Source: CAD feature listing. Evaluate the final solid. Frame: model axes, mm. A direction names the side the tool comes from. Give positions to 0.01 mm unless a question says otherwise; leave off trailing zeros. Loops run counter-clockwise (first coordinate to the right, second up) from the corner with the lowest first, then second, coordinate; pieces in that order, holes last. Notation, with made-up numbers: M 18,65 L 41,65 A15 cw 41,75 Z; hole C -16.5,-4 d10. An arc over 180 degrees is marked long. Answer in a Markdown table with one row per item.
```python
from build123d import *

# Parameters (mm, degrees)
BOSS_EXTRUDE1_DEPTH      = 1.5875
BOSS_EXTRUDE1_DEPTH_BACK = 1.5875
SKETCH1_W                = 255.27
SKETCH1_H                = 73.96988
SKETCH1_R                = 1.5
BOSS_EXTRUDE2_DEPTH      = 1.5875
BOSS_EXTRUDE2_DEPTH_BACK = 1.5875
SKETCH1_4_W              = 255.27
SKETCH1_4_H              = 73.96988
CUT_EXTRUDE1_DEPTH       = 1.5875
CUT_EXTRUDE2_DEPTH       = 3.175
CUT_EXTRUDE2_DEPTH_BACK  = 3.175
SKETCH1_6_R              = 1.5
SKETCH3_R                = 1.5875
BOSS_EXTRUDE3_DEPTH      = 3.175


with BuildPart() as part:
    # Sketch1 → Boss-Extrude1 (new, two sides: drawn at the far end of the back side and taken through both)
    with BuildSketch(Plane(origin=(0, 0, 0), x_dir=(1, 0, 0), z_dir=(0, 1, 0)).offset(-BOSS_EXTRUDE1_DEPTH_BACK)):
        with Locations((127.635, 36.98494)):
            Rectangle(SKETCH1_W, SKETCH1_H)
        with Locations(Location((178.435, 68.57238, 0), (0, 0, 270))):
            Circle(SKETCH1_R, mode=Mode.SUBTRACT)
        with Locations(Location((178.435, 5.3975, 0), (0, 0, 270))):
            Circle(SKETCH1_R, mode=Mode.SUBTRACT)
        with Locations(Location((229.235, 68.57238, 0), (0, 0, 270))):
            Circle(SKETCH1_R, mode=Mode.SUBTRACT)
        with Locations(Location((229.235, 5.3975, 0), (0, 0, 270))):
            Circle(SKETCH1_R, mode=Mode.SUBTRACT)
        with Locations(Location((127.635, 68.57238, 0), (0, 0, 270))):
            Circle(SKETCH1_R, mode=Mode.SUBTRACT)
        with Locations(Location((127.635, 5.3975, 0), (0, 0, 270))):
            Circle(SKETCH1_R, mode=Mode.SUBTRACT)
        with Locations(Location((26.035, 5.3975, 0), (0, 0, 270))):
            Circle(SKETCH1_R, mode=Mode.SUBTRACT)
        with Locations(Location((76.835, 5.3975, 0), (0, 0, 270))):
            Circle(SKETCH1_R, mode=Mode.SUBTRACT)
        with Locations(Location((26.035, 68.57238, 0), (0, 0, 270))):
            Circle(SKETCH1_R, mode=Mode.SUBTRACT)
        with Locations(Location((76.835, 68.57238, 0), (0, 0, 270))):
            Circle(SKETCH1_R, mode=Mode.SUBTRACT)
    extrude(amount=BOSS_EXTRUDE1_DEPTH + BOSS_EXTRUDE1_DEPTH_BACK)

    # Sketch1_4 → Boss-Extrude2 (add, two sides: drawn at the far end of the back side and taken through both)
    with BuildSketch(Plane(origin=(0, 0, 0), x_dir=(1, 0, 0), z_dir=(0, 1, 0)).offset(-BOSS_EXTRUDE2_DEPTH_BACK)):
        with Locations((127.635, 36.98494)):
            Rectangle(SKETCH1_4_W, SKETCH1_4_H)
    extrude(amount=BOSS_EXTRUDE2_DEPTH + BOSS_EXTRUDE2_DEPTH_BACK)

    # Sketch2 → Cut-Extrude1 (cut)
    with BuildSketch(Plane(origin=(0, 1.5875, 0), x_dir=(1, 0, 0), z_dir=(0, 1, 0))):
        with BuildLine():
            Line((13.335, 63.80988), (241.935, 63.80988))
            ThreePointArc((241.935, 63.80988), (244.18006403, 62.87994403), (245.11, 60.63488))
            Line((245.11, 60.63488), (245.11, 13.335))
            ThreePointArc((245.11, 13.335), (244.18006403, 11.08993597), (241.935, 10.16))
            Line((241.935, 10.16), (13.335, 10.16))
            ThreePointArc((13.335, 10.16), (11.08993597, 11.08993597), (10.16, 13.335))
            Line((10.16, 13.335), (10.16, 60.63488))
            ThreePointArc((10.16, 60.63488), (11.08993597, 62.87994403), (13.335, 63.80988))
        make_face()
    extrude(amount=-CUT_EXTRUDE1_DEPTH, mode=Mode.SUBTRACT)

    # Sketch1_6 → Cut-Extrude2 (cut, two sides: drawn at the far end of the back side and taken through both)
    with BuildSketch(Plane(origin=(0, 0, 0), x_dir=(1, 0, 0), z_dir=(0, 1, 0)).offset(-CUT_EXTRUDE2_DEPTH_BACK)):
        with Locations(Location((178.435, 68.57238, 0), (0, 0, 270))):
            Circle(SKETCH1_6_R)
        with Locations(Location((178.435, 5.3975, 0), (0, 0, 270))):
            Circle(SKETCH1_6_R)
        with Locations(Location((229.235, 68.57238, 0), (0, 0, 270))):
            Circle(SKETCH1_6_R)
        with Locations(Location((229.235, 5.3975, 0), (0, 0, 270))):
            Circle(SKETCH1_6_R)
        with Locations(Location((127.635, 68.57238, 0), (0, 0, 270))):
            Circle(SKETCH1_6_R)
        with Locations(Location((127.635, 5.3975, 0), (0, 0, 270))):
            Circle(SKETCH1_6_R)
        with Locations(Location((26.035, 5.3975, 0), (0, 0, 270))):
            Circle(SKETCH1_6_R)
        with Locations(Location((76.835, 5.3975, 0), (0, 0, 270))):
            Circle(SKETCH1_6_R)
        with Locations(Location((26.035, 68.57238, 0), (0, 0, 270))):
            Circle(SKETCH1_6_R)
        with Locations(Location((76.835, 68.57238, 0), (0, 0, 270))):
            Circle(SKETCH1_6_R)
    extrude(amount=CUT_EXTRUDE2_DEPTH + CUT_EXTRUDE2_DEPTH_BACK, mode=Mode.SUBTRACT)

    # Sketch3 → Boss-Extrude3 (add)
    # profile 1 of 4: a face of its own
    with BuildSketch(Plane.XZ.offset(1.5875)):
        with BuildLine():
            Line((0, -17.4625), (0, 0))
            Line((0, 0), (-7.9375, 0))
            ThreePointArc((-7.9375, 0), (-11.305096045, -1.394903955), (-12.7, -4.7625))
            Line((-12.7, -4.7625), (-12.7, -7.9375))
            ThreePointArc((-12.7, -7.9375), (-11.305096045, -11.305096045), (-7.9375, -12.7))
            Line((-7.9375, -12.7), (-4.7625, -12.7))
            ThreePointArc((-4.7625, -12.7), (-1.394903955, -14.094903955), (0, -17.4625))
        make_face()
        with Locations(Location((-6.35, -6.35, 0), (0, 0, 270))):
            Circle(SKETCH3_R, mode=Mode.SUBTRACT)
    # profile 2 of 4: a face of its own
    with BuildSketch(Plane.XZ.offset(1.5875)):
        with BuildLine():
            Line((-7.9375, -61.26988), (-4.7625, -61.26988))
            ThreePointArc((-4.7625, -61.26988), (-1.394903955, -59.874976045), (0, -56.50738))
            Line((0, -56.50738), (0, -73.96988))
            Line((0, -73.96988), (-7.9375, -73.96988))
            ThreePointArc((-7.9375, -73.96988), (-11.305096045, -72.574976045), (-12.7, -69.20738))
            Line((-12.7, -69.20738), (-12.7, -66.03238))
            ThreePointArc((-12.7, -66.03238), (-11.305096045, -62.664783955), (-7.9375, -61.26988))
        make_face()
        with Locations(Location((-6.35, -67.61988, 0), (0, 0, 270))):
            Circle(SKETCH3_R, mode=Mode.SUBTRACT)
    # profile 3 of 4: a face of its own
    with BuildSketch(Plane.XZ.offset(1.5875)):
        with BuildLine():
            Line((255.27, -56.50738), (255.27, -73.96988))
            Line((255.27, -73.96988), (263.2075, -73.96988))
            ThreePointArc((263.2075, -73.96988), (266.575096045, -72.574976045), (267.97, -69.20738))
            Line((267.97, -69.20738), (267.97, -66.03238))
            ThreePointArc((267.97, -66.03238), (266.575096045, -62.664783955), (263.2075, -61.26988))
            Line((263.2075, -61.26988), (260.0325, -61.26988))
            ThreePointArc((260.0325, -61.26988), (256.664903955, -59.874976045), (255.27, -56.50738))
        make_face()
        with Locations(Location((261.62, -67.61988, 0), (0, 0, 270))):
            Circle(SKETCH3_R, mode=Mode.SUBTRACT)
    # profile 4 of 4: a face of its own
    with BuildSketch(Plane.XZ.offset(1.5875)):
        with BuildLine():
            Line((263.2075, -12.7), (260.0325, -12.7))
            ThreePointArc((260.0325, -12.7), (256.664903955, -14.094903955), (255.27, -17.4625))
            Line((255.27, -17.4625), (255.27, 0))
            Line((255.27, 0), (263.2075, 0))
            ThreePointArc((263.2075, 0), (266.575096045, -1.394903955), (267.97, -4.7625))
            Line((267.97, -4.7625), (267.97, -7.9375))
            ThreePointArc((267.97, -7.9375), (266.575096045, -11.305096045), (263.2075, -12.7))
        make_face()
        with Locations(Location((261.62, -6.35, 0), (0, 0, 270))):
            Circle(SKETCH3_R, mode=Mode.SUBTRACT)
    extrude(amount=-BOSS_EXTRUDE3_DEPTH)


solid = part.part
```
1) Set-up query: faces 1 (the flat face through (129, 0, -37)), 2 (the cylindrical face through (-11.27, -0.02, -72.61)), 3 (the cylindrical face through (-11.27, -0.02, -1.36)), 4 (the cylindrical face through (266.61, -0.02, -11.27)), 5 (the cylindrical face through (-1.43, -0.02, -14.06)). Return all of +Z, -Z, +X, -X, +Y, -Y with unobstructed straight access to the full face (end or side cutting, diameter ignored); none if empty.
Reply:
| item | result |
|---|---|
| face 1 | +Y |
| face 2 | -Z, -X, +Y, -Y |
| face 3 | +Z, -X, +Y, -Y |
| face 4 | +X, +Y, -Y |
| face 5 | -X, +Y, -Y |
2) Section A-A, the plane z = -32. Return loops of the section in (x, y).
Reply:
| item | result |
|---|---|
| outline | M 0,-1.59 L 255.27,-1.59 L 255.27,1.59 L 245.11,1.59 L 245.11,0 L 10.16,0 L 10.16,1.59 L 0,1.59 Z |
3) Section C-C, the plane y = 0.8. Count the separate pieces of the cut face and the enclosed holes in it, then the cut area to 3 significant figures.
Reply:
| item | result |
|---|---|
| separate pieces | 1 |
| enclosed holes | 15 |
| area | 6,810 mm² |
4) Section B-B, the plane x = 218.5. Return loops of the section in (y, z), then the cut area to 3 significant figures.
Reply:
| item | result |
|---|---|
| outline | M -1.59,-73.97 L 1.59,-73.97 L 1.59,-63.81 L 0,-63.81 L 0,-10.16 L 1.59,-10.16 L 1.59,0 L -1.59,0 Z |
| area | 150 mm² |
5) Pull-direction query (Z, two-part tool) for faces 6 (the cylindrical face through (266.54, -0.02, -72.61)), 7 (the cylindrical face through (256.7, -0.02, -14.06)), 8 (the flat face through (126, -1.588, -36)), 9 (the cylindrical face through (266.54, -0.02, -1.36)); classes: released by +Z, released by -Z, zero draft, split by the parting line, or undercut.
Reply:
| item | result |
|---|---|
| face 6 | released by -Z |
| face 7 | undercut |
| face 8 | zero draft |
| face 9 | released by +Z |
6) Material intervals for L1, parallel to Z at x = 137, y = 1.1; L2, parallel to X at y = 0.4, z = -48; L3, parallel to X at y = -0.2, z = -7.5, sorted ascending.
Reply:
| item | result |
|---|---|
| L1 | z = -73.97 to -63.81, -10.16 to 0 |
| L2 | x = 0 to 10.16, 245.11 to 255.27 |
| L3 | x = -12.7 to -7.44, -5.26 to 260.53, 262.71 to 267.97 |
7) Pin query (flat end, axial travel): pin 1 Ø2 at (x, z) = (130, -18.5) entering from +Y; pin 2 Ø1.3 at (y, z) = (0.5, -27) entering from -X. Return the tip coordinate at first contact, or that it passes through.
Reply:
| item | result |
|---|---|
| pin 1 | stops at y = 0 |
| pin 2 | stops at x = 0 |
